```python
from build123d import *

# Parameters (mm, degrees)
SKETCH2_W          = 32
SKETCH2_H          = 32
CUT_EXTRUDE1_DEPTH = 9.4


with BuildPart() as part:
    # Sketch1 → Revolve1 (revolve)
    with BuildSketch(Plane(origin=(0, 0, 0), x_dir=(1, 0, 0), z_dir=(0, 1, 0))):
        Polygon((0, 0), (-8, 0), (-9.6, 0.923760431), (-9.6, 8.476239569), (-8, 9.4), (-5, 9.4), (-5, 10.4), (-6, 11.4), (-6, 20.3865), (-5.3865, 21), (-3.3, 21), (-3.3, 21.2), (-3, 21.2), (-3, 21.8), (-3.2, 22), (-4.95, 22), (-4.95, 23.3), (-4.75, 23.5), (0, 23.5), align=None)
    revolve(axis=Axis((0, 0, -23.5), (0, 0, 1)))

    # Sketch2 → Cut-Extrude1 (cut)
    with BuildSketch(Plane.XY):
        Rectangle(SKETCH2_W, SKETCH2_H)
        Polygon((-9.237604307, 0), (-4.618802154, -8), (4.618802154, -8), (9.237604307, 0), (4.618802154, 8), (-4.618802154, 8), align=None, mode=Mode.SUBTRACT)
    extrude(amount=-CUT_EXTRUDE1_DEPTH, mode=Mode.SUBTRACT)

    # Sketch3 → Cut-Revolve1 (revolve, cut)
    with BuildSketch(Plane(origin=(0, 0, 0), x_dir=(0, 0, -1), z_dir=(1, 0, 0))):
        Polygon((0, 0), (0, 4.864), (0.581, 4.283), (8.4, 4.283), (8.4, 1.5), (10, 1.5), (10.5, 2), (23.2, 2), (23.5, 2.3), (23.5, 0), align=None)
    revolve(axis=Axis((0, 0, -23.5), (0, 0, 1)), mode=Mode.SUBTRACT)


solid = part.part
```
Read the model definition and answer for the solid it produces. Units are mm, in the model's axes. A direction names the side the tool comes from. Coordinates: 2 decimals unless noted, no trailing zeros. Write each loop counter-clockwise with the first axis right and the second up, starting at its lowest first coordinate (ties: lowest second). Pieces come first, ordered by that corner, then holes. Notation, with made-up numbers: (59, -11) -> (72, -11) arc R13 ccw to (72, 5) -> close; hole circle Ø6 at (40, 26.25). An arc over 180 degrees is marked (long way). Return JSON: item names as keys, results as strings.
1. Determine the mould class of faces 4 (the face through (-4.17, -7.17, -9.23)), 5 (the face through (-4.13, 7.19, -9.23)), 6 (the face through (-1.286, 4.085, -4.545)) for opening direction Y: pulls with the +Y half, pulls with the -Y half, needs draft (parallel to the pull), parting line crosses it, or undercut.
Found:
{"face 4": "pulls with the -Y half", "face 5": "pulls with the +Y half", "face 6": "undercut"}
2. Each of these flat-tipped pins is pushed along its axis until it touches: P1, Ø2, axis at x = -6, y = -5, coming from the -Z side; P2, Ø4.5, axis at x = 0, y = 0, coming from the +Z side; P3, Ø3, axis at y = 5.5, z = -17, coming from the -X side. Where does it stop, or does it pass through?
Found:
{"P1": "z = -9.4", "P2": "z = -8.4", "P3": "x = -4.47"}
3. A tool of negligible diameter and unlimited length cuts with its end or side. For faces 1 (the face through (0, -8, -5)), 2 (the face through (0, 4, -21)), 3 (the face through (-4.72, -1.49, -22.66)), from which of +Z, -Z, +X, -X, +Y, -Y can it reach the whole face along a straight path? Write none if from no direction.
Found:
{"face 1": "+Z, -Z, +X, -X, -Y", "face 2": "none", "face 3": "-Z"}
4. Find the intervals of material crossed by line 1 along Y through (x, z) = (0, -9.6); line 2 along X through (y, z) = (0, -18.5); line 3 along Z through (x, y) = (-4.25, 5.25), in increasing order. Write a range as from..to.
Found:
{"line 1": "-5..-1.5, 1.5..5", "line 2": "-6..-2, 2..6", "line 3": "-9.4..0"}
5. A cutting plane is placed at A-A (z = -17.5). Determine the outline of the cut face in (x, y), and give its area (3 significant figures).
Found:
{"outline": "circle Ø12 at (0, 0); hole circle Ø4 at (0, 0)", "area": "101 mm2"}
